Part model, mm, in its own coordinate system. A direction names the side the tool comes from. Round coordinates to 2 decimals unless told otherwise and drop trailing zeros. Write each loop counter-clockwise with the first axis right and the second up, starting at its lowest first coordinate (ties: lowest second). Pieces come first, ordered by that corner, then holes. Notation, with made-up numbers: M 8,13 L 42,13 A21 cw 42,24 Z; hole C 73.5,-35 d10. An arc over 180 degrees is marked long. Use one line per item in the form item = value. Start each with the question number.
Item 1: Probe L1, parallel to Y at x = -4.5, z = -10; L2, parallel to X at y = 2, z = -5; L3, parallel to X at y = 12.5, z = -16.5. List the from-to ranges inside material, lowest first.
Item 2: Flat gauge pins, fed straight in: pin 1 Ø1 at (y, z) = (7.5, -16.5) entering from +X; pin 2 Ø2.5 at (y, z) = (8, -10) entering from +X; pin 3 Ø3 at (y, z) = (6, -7) entering from -X; pin 4 Ø4.5 at (x, y) = (-7.5, 7.5) entering from +Z. Where does each tip first touch, or does it go through?
Item 3: Mould opens along Z. For faces 6 (the face through (-6, 1, 0)), 7 (the face through (-12, 1, -10)), 8 (the face through (-6, 1, -17)), 9 (the face through (-6, 8, -19)) say: +Z half, -Z half, draft (parallel to the pull), parting line (faces both ways), or undercut.
Item 4: Cut at A-A, the plane z = -10. Give the cut face in (x, y).
Item 5: Which spindle directions (+Z, -Z, +X, -X, +Y, -Y) get a long thin tool onto all of the face, cutting with end or side? Do faces 1 (the face through (-1, 9.34, -12.01)), 2 (the face through (-2.1, 1.52, -3.57)), 3 (the face through (-5.93, 9.52, -8.34)), 4 (the face through (-0.57, 1.52, -19.4)), 5 (the face through (-11, 9.34, -7.99)). Say none if no direction does.
Item 6: Cut at D-D, the plane z = -13.5. Give the cut face in (x, y).
Item 7: Cut at C-C, the plane x = -6.75. Give the cut face in (y, z).
Item 8: Cut at B-B, the plane y = 8. Give the cut face in (x, z).
Autodesk Inventor part; units mm, degrees
ref_plane "YZ Plane" through (0, 0, 0) normal (1, 0, 0) x (0, 1, 0)
ref_plane "XZ Plane" through (0, 0, 0) normal (0, 1, 0) x (-1, 0, 0)
ref_plane "XY Plane" through (0, 0, 0) normal (0, 0, 1) x (1, 0, 0)
sketch "Sketch1" plane through (0, 0, 0) normal (0, 1, 0) x (-1, 0, 0)
  line L0 (0, 0) -> (12, 0)
  line L1 (12, 0) -> (12, -20)
  line L2 (12, -20) -> (0, -20)
  line L3 (0, -20) -> (0, 0)
  dimension "d0" = 12
  dimension "d1" = 20
extrude "Extrusion1" add sketch "Sketch1" along normal blind 3
sketch "Sketch2" plane through (0, 3, 0) normal (0, 1, 0) x (1, 0, 0)
  line L0 (-12, 20) -> (-12, 0) construction
  line L1 (-12, 10) -> (0, 10) construction
  line L2 (0, 0) -> (0, 20) construction
  line L3 (-1, 1) -> (-11, 1) construction
  line L4 (-11, 1) -> (-11, 19) construction
  line L5 (-11, 19) -> (-1, 19) construction
  line L6 (-1, 19) -> (-1, 1) construction
  line L7 (-1, 1) -> (-11, 19) construction
  line L8 (-11, 1) -> (-1, 19) construction
  line L9 (-1, 1) -> (-11, 1)
  line L10 (-11, 1) -> (-11, 19)
  line L11 (-11, 19) -> (-1, 19)
  line L12 (-1, 19) -> (-1, 1)
  line L13 (-1, 1) -> (-11, 19) construction
  line L14 (-11, 1) -> (-1, 19) construction
  point P0 (-6, 10)
  point P1 (-6, 10)
  dimension "d4" = 10
  dimension "d5" = 18
extrude "Extrusion2" add sketch "Sketch2" along normal blind 11
sketch "Sketch3" plane through (-1, 3, -1) normal (1, 0, 0) x (0, 0, -1)
  line L0 (19, -3) -> (-1, -3) construction
  line L1 (9, -3) -> (9, 5) construction
  circle A0 centre (9, 5) radius 2.25
  dimension "d8" = 8
  dimension "d9" = 4.5
extrude "Extrusion3" cut sketch "Sketch3" against normal blind 10
sketch "Sketch4" plane through (0, 0, 0) normal (0, -1, 0) x (1, 0, 0)
  line L0 (0, 0) -> (0, -20) construction
  line L1 (0, -10) -> (-12, -10) construction
  line L2 (-12, -20) -> (-12, 0) construction
  line L3 (-10.5, -3) -> (-1.5, -3) construction
  line L4 (-1.5, -3) -> (-1.5, -17) construction
  line L5 (-1.5, -17) -> (-10.5, -17) construction
  line L6 (-10.5, -17) -> (-10.5, -3) construction
  line L7 (-10.5, -3) -> (-1.5, -17) construction
  line L8 (-1.5, -3) -> (-10.5, -17) construction
  line L9 (-1.5, -3) -> (-10.5, -3) construction
  line L10 (-10.5, -3) -> (-10.5, -17) construction
  line L11 (-10.5, -17) -> (-1.5, -17) construction
  line L12 (-1.5, -17) -> (-1.5, -3) construction
  line L13 (-1.5, -3) -> (-10.5, -3)
  line L14 (-10.5, -3) -> (-10.5, -17)
  line L15 (-10.5, -17) -> (-1.5, -17)
  line L16 (-1.5, -17) -> (-1.5, -3)
  point P0 (-6, -10)
  dimension "d12" = 9
  dimension "d13" = 14
extrude "Extrusion4" cut sketch "Sketch4" against normal blind 3
fillet "Fillet1" radius 2 8 edges at (-1.5, 1.5, -3) (-1.5, 1.5, -17) (-10.5, 1.5, -3) (-10.5, 1.5, -17) (0, 1.5, 0) (0, 1.5, -20) (-12, 1.5, 0) (-12, 1.5, -20)
chamfer "Chamfer1" distance 0.5 angle 45 8 edges at (-1, 8.5, -1) (-11, 14, -10) (-1, 8.5, -19) (-11, 8.5, -19) (-11, 8.5, -1) (-6, 14, -1) (-6, 14, -19) (-1, 14, -10)
properties part number "Steam Chest Slide Valve" material "Brass, Soft Yellow"
Model answer:
q1.L1 = 3 to 5.75, 10.25 to 14
q1.L2 = -12 to -10.5, -1.5 to 0
q1.L3 = -11 to -1
q2.pin_1 = -1
q2.pin_2 = through
q2.pin_3 = -11
q2.pin_4 = -1
q3.face_6 = +Z half
q3.face_7 = draft
q3.face_8 = undercut
q3.face_9 = -Z half
q4.outline = M -12,0 L -10.5,0 L -10.5,3 L -1.5,3 L -1.5,0 L 0,0 L 0,3 L -1,3 L -1,5.75 L -11,5.75 L -11,3 L -12,3 Z; M -11,10.25 L -1,10.25 L -1,13.5 L -1.5,14 L -10.5,14 L -11,13.5 Z
q5.face_1 = +Z, -Z, +X, +Y
q5.face_2 = -Y
q5.face_3 = +X, -X
q5.face_4 = -Z, +X, +Y, -Y
q5.face_5 = +Z, -Z, -X, +Y
q6.outline = M -12,0 L -10.5,0 L -10.5,3 L -1.5,3 L -1.5,0 L 0,0 L 0,3 L -1,3 L -1,13.5 L -1.5,14 L -10.5,14 L -11,13.5 L -11,3 L -12,3 Z
q7.outline = M 0,-20 L 3,-20 L 3,-19 L 13.5,-19 L 14,-18.5 L 14,-1.5 L 13.5,-1 L 3,-1 L 3,0 L 0,0 L 0,-3 L 3,-3 L 3,-17 L 0,-17 Z; hole C 8,-10 d4.5
q8.outline = M -11,-18.5 L -10.5,-19 L -1.5,-19 L -1,-18.5 L -1,-12.25 L -11,-12.25 Z; M -11,-7.75 L -1,-7.75 L -1,-1.5 L -1.5,-1 L -10.5,-1 L -11,-1.5 Z
